The model under review builds one solid part; all positions refer to its coordinate system, in mm. A direction names the side the tool comes from. Round coordinates to 2 decimals unless told otherwise and drop trailing zeros. Write each loop counter-clockwise with the first axis right and the second up, starting at its lowest first coordinate (ties: lowest second). Pieces come first, ordered by that corner, then holes.
Item 1: Add section B-B (z = 13.5). Give the boundary of the cut face in (x, y).
Item 2: Machinability: for faces 4 (the face through (-6.31, -203.42, -5.92)), 5 (the face through (15, -191, 0)), 6 (the face through (-53.115, -230.351, 46.084)), 7 (the face through (-75, -243, 40)), which of the approach directions +Z, -Z, +X, -X, +Y, -Y give a long, thin tool a straight path to every point of the face, cutting with its end or side? Answer none if there is none.
Item 3: Add section A-A (z = 46). Give the boundary of the cut face in (x, y), plus the area to 3 significant figures.
Item 4: To check wall thickness, follow L1, parallel to X at y = -233, z = 6.5; L2, parallel to X at y = -238, z = -5.5; L3, parallel to Y at x = -1.5, z = 31. State the ranges of each line that lie inside material, in increasing order.
Item 5: Add section C-C (x = 13). Give the boundary of the cut face in (y, z), plus the area to 3 significant figures.
Item 6: Clearance check with flat-ended pins moving along their axes: pin 1 Ø8 at (y, z) = (-234.5, 39) entering from +X; pin 2 Ø7 at (x, y) = (-42, -224) entering from -Z; pin 3 Ø7 at (x, y) = (-41.5, -226.5) entering from +Z. State where each tip first meets the part, or that it passes through.
Item 7: Draft analysis for pull direction X (two halves, no side actions). For faces 1 (the face through (-45, -226, 40)), 2 (the face through (9.24, -194.35, -5.92)), 3 (the face through (-6.31, -203.42, 46.08)), state which applies: +X half, -X half, draft (parallel to the pull), parting line (faces both ways), or undercut.
Item 8: Add section D-D (z = 7). Give the boundary of the cut face in (x, y), plus the area to 3 significant figures.
```python
from build123d import *

# Parameters (mm, degrees)
BOSS_EXTRU_1_DEPTH      = 40
BOSS_EXTRU_2_DEPTH      = 12
BOSS_EXTRU_2_DEPTH_BACK = 52
ESQUISSE2_R             = 10
ENL_V_MAT_EXTRU_2_DEPTH = 12


with BuildPart() as part:
    # Esquisse1 → Boss.-Extru.1 (new body)
    with BuildSketch(Plane.XY):
        Polygon((-82.421937441, -243.855765017), (20, -184.722431864), (23, -189.918584287), (-79.421937441, -249.05191744), align=None)
    extrude(amount=BOSS_EXTRU_1_DEPTH)

    # Esquisse3 → Boss.-Extru.2 (add, two sides: drawn at the far end of the back side and taken through both)
    with BuildSketch(Plane(origin=(0, 0, 0), x_dir=(-1, 0, 0), z_dir=(0, 0, -1)).offset(-BOSS_EXTRU_2_DEPTH_BACK)):
        Polygon((4.828282819, -205.985250863), (7.828282819, -200.789098441), (-7.76017445, -191.789098441), (-10.76017445, -196.985250863), align=None)
        Polygon((39.005197355, -218.789098441), (31.210968721, -214.289098441), (28.210968721, -219.485250863), (36.005197355, -223.985250863), align=None)
        Polygon((28.210968721, -219.485250863), (31.210968721, -214.289098441), (23.416740087, -209.789098441), (20.416740087, -214.985250863), align=None)
        Polygon((70.182111891, -236.789098441), (54.593654623, -227.789098441), (51.593654623, -232.985250863), (67.182111891, -241.985250863), align=None)
    extrude(amount=BOSS_EXTRU_2_DEPTH + BOSS_EXTRU_2_DEPTH_BACK)

    # Esquisse2 → Enlèv. mat.-Extru.2 (cut)
    with BuildSketch(Plane(origin=(84.987159322, -147.202077936, 0), x_dir=(0.8660254037844385, 0.5000000000000003, 0), z_dir=(-0.5000000000000003, 0.8660254037844385, 0))):
        with Locations(Location((-164.174041009, -20, 0), (0, 0, 180))):
            Circle(ESQUISSE2_R)
        with Locations(Location((-104.174041009, -20, 0), (0, 0, 180))):
            Circle(ESQUISSE2_R)
    extrude(amount=-ENL_V_MAT_EXTRU_2_DEPTH, mode=Mode.SUBTRACT)


solid = part.part
```
Numbers:
1. outline: (-82.42, -243.86) - (-79.42, -249.05) - (-60.77, -238.28) - (-63.77, -233.09) - close; (-50.61, -225.49) - (-47.61, -230.69) - (-8.81, -208.28) - (-11.81, -203.09) - close; (1.35, -195.49) - (4.35, -200.69) - (23, -189.92) - (20, -184.72) - close
2. face 4: -Z, -X, -Y
2. face 5: -Z, +X, +Y
2. face 6: +Z, +X, +Y
2. face 7: +Z, -X, -Y
3. outline: (-70.18, -236.79) - (-67.18, -241.99) - (-51.59, -232.99) - (-54.59, -227.79) - close; (-39.01, -218.79) - (-36.01, -223.99) - (-20.42, -214.99) - (-23.42, -209.79) - close; (-7.83, -200.79) - (-4.83, -205.99) - (10.76, -196.99) - (7.76, -191.79) - close
3. area: 324 mm2
4. L1: x = -63.62 to -51.62
4. L2: x = -69.48 to -60.28
4. L3: y = -204.06 to -197.14
5. outline: (-195.69, 0) - (-188.76, 0) - (-188.76, 40) - (-195.69, 40) - close
5. area: 277 mm2
6. pin 1: stops at x = -47.29
6. pin 2: stops at z = 0
6. pin 3: stops at z = 40
7. face 1: draft
7. face 2: +X half
7. face 3: -X half
8. outline: (-82.42, -243.86) - (-79.42, -249.05) - (23, -189.92) - (20, -184.72) - close
8. area: 710 mm2
